Design review of the part built by this model. Coordinates are the model's own, in mm. Face numbers are marked on the shaded views. Round coordinates to 2 decimals unless told otherwise and drop trailing zeros. Order: outer loops, then holes, each group sorted by start corner. A loop starts at its lowest first (then second) coordinate and runs counter-clockwise, first axis right, second up. Notation, with made-up numbers: M 76.25,-32.5 L 113.25,-32.5 A30 cw 113.25,-1.5 Z; hole C 74,11 d1. An arc over 180 degrees is marked long. Write item = value, one per line. Start each with the question number.
```python
from build123d import *

# Parameters (mm, degrees)
F1_DEPTH = 2600
F2_W     = 560
F2_H     = 1279.0293264389
F3_DEPTH = 95.001
F4_W     = 765
F4_H     = 2300
F5_DEPTH = 95.001
F6_R     = 3


with BuildPart() as f1:
    # F0 (on Top) → F1 (new body)
    with BuildSketch(Plane.XY):
        Polygon((-271.6449069816, 555.1264761336), (-271.6449069816, -244.8735238664), (-176.6449069816, -244.8735238664), (-176.6449069816, 460.1264761336), (728.3550930184, 460.1264761336), (728.3550930184, 555.1264761336), align=None)
        Polygon((-259.1449069816, 542.6264761336), (715.8550930184, 542.6264761336), (715.8550930184, 472.6264761336), (-189.1449069816, 472.6264761336), (-189.1449069816, -232.3735238664), (-259.1449069816, -232.3735238664), align=None, mode=Mode.SUBTRACT)
    extrude(amount=F1_DEPTH)

    # F2 (on face) → F3 (cut, through all)
    with BuildSketch(Plane.YZ.offset(-176.6449069816)):
        with Locations((107.6264761336, 1660.4853367805)):
            Rectangle(F2_W, F2_H)
    extrude(amount=-F3_DEPTH, mode=Mode.SUBTRACT)

    # F4 (on face) → F5 (cut, through all)
    with BuildSketch(Plane.XZ.offset(-460.1264761336)):
        with Locations((275.8550930184, 1150)):
            Rectangle(F4_W, F4_H)
    extrude(amount=-F5_DEPTH, mode=Mode.SUBTRACT)

    # F6
    f6_edges = [f1.edges().sort_by_distance(p)[0] for p in [
        (-106.644907, 542.626476, 1150),
        (-106.644907, 548.876476, 0),
        (-106.644907, 555.126476, 1150),
        (-106.644907, 548.876476, 2300),
        (-106.644907, 460.126476, 1150),
        (-106.644907, 466.376476, 0),
        (-106.644907, 472.626476, 1150),
        (-106.644907, 466.376476, 2300),
        (275.855093, 542.626476, 2300),
        (275.855093, 555.126476, 2300),
        (658.355093, 548.876476, 2300),
        (275.855093, 460.126476, 2300),
        (275.855093, 472.626476, 2300),
        (658.355093, 466.376476, 2300),
        (-259.144907, 107.626476, 2300),
        (-265.394907, -172.373524, 2300),
        (-271.644907, 107.626476, 2300),
        (-265.394907, 387.626476, 2300),
        (-176.644907, 107.626476, 2300),
        (-182.894907, -172.373524, 2300),
        (-189.144907, 107.626476, 2300),
        (-182.894907, 387.626476, 2300),
        (-259.144907, 387.626476, 1660.485337),
        (-271.644907, 387.626476, 1660.485337),
        (-265.394907, 387.626476, 1020.970674),
        (-176.644907, 387.626476, 1660.485337),
        (-189.144907, 387.626476, 1660.485337),
        (-182.894907, 387.626476, 1020.970674),
        (-271.644907, -172.373524, 1660.485337),
        (-271.644907, 107.626476, 1020.970674),
        (658.355093, 555.126476, 1150),
        (-259.144907, -172.373524, 1660.485337),
        (-259.144907, 107.626476, 1020.970674),
        (658.355093, 542.626476, 1150),
        (-189.144907, -172.373524, 1660.485337),
        (-189.144907, 107.626476, 1020.970674),
        (658.355093, 472.626476, 1150),
        (658.355093, 460.126476, 1150),
        (-176.644907, 107.626476, 1020.970674),
        (-176.644907, -172.373524, 1660.485337),
    ]]
    fillet(f6_edges, radius=F6_R)


solid = f1.part
```
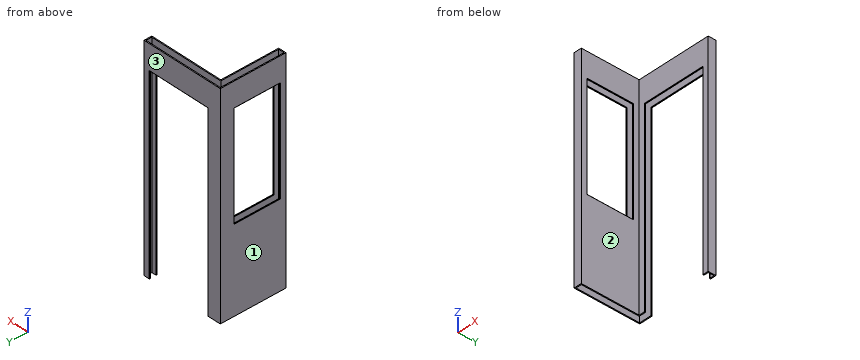
(1) Insertion check: pin 1 (2 mm diameter, centred on x = -265, y = 182.5, fed in from -Z); pin 2 (12 mm diameter, centred on y = 451.5, z = 1249, fed in from +X). Each pin has a flat end and moves straight along its axis. Give the tip position at first contact, or say it passes through.
(2) Consider section A-A, the plane x = -143. Write out the cut boundary in (y, z).
(3) For line 1 along Y through (x, z) = (-185.5, 1941); line 2 along Y through (x, z) = (636, 2445.5); line 3 along X through (y, z) = (483.5, 499), list the stretches that pass through material, from the lowest coordinate up. Write a range as [from, to].
(4) Consider section C-C, the plane z = 590.5. Write out the cut boundary in (x, y).
(5) Consider section B-B, the plane y = 161.5. Write out the cut boundary in (x, z).
(6) Draft analysis for pull direction X (two halves, no side actions). For the marked faces 1, 2 and 3, state which applies: pulls with the +X half, pulls with the -X half, needs draft (parallel to the pull), parting line crosses it, or undercut.
(7) Consider section D-D, the plane x = 426. Write out the cut boundary in (y, z), then the cut area to 3 significant figures.
Completed:
q1.pin_1 = 0
q1.pin_2 = -176.64
q2.outline = M 460.13,0 L 472.63,0 L 472.63,2600 L 460.13,2600 Z; M 542.63,0 L 555.13,0 L 555.13,2600 L 542.63,2600 Z
q3.line_1 = [-244.87, -172.37], [387.63, 472.63], [542.63, 555.13]
q3.line_2 = [460.13, 472.63], [542.63, 555.13]
q3.line_3 = [-271.64, -259.14], [715.86, 728.36]
q4.outline = M -271.64,-244.87 L -176.64,-244.87 L -176.64,460.13 L -109.64,460.13 A3 ccw -106.64,463.13 L -106.64,469.63 A3 ccw -109.64,472.63 L -189.14,472.63 L -189.14,-232.37 L -259.14,-232.37 L -259.14,542.63 L -109.64,542.63 A3 ccw -106.64,545.63 L -106.64,552.13 A3 ccw -109.64,555.13 L -271.64,555.13 Z; M 658.36,463.13 A3 ccw 661.36,460.13 L 728.36,460.13 L 728.36,555.13 L 661.36,555.13 A3 ccw 658.36,552.13 L 658.36,545.63 A3 ccw 661.36,542.63 L 715.86,542.63 L 715.86,472.63 L 661.36,472.63 A3 ccw 658.36,469.63 Z
q5.outline = M -271.64,0 L -259.14,0 L -259.14,1017.97 A3 ccw -262.14,1020.97 L -268.64,1020.97 A3 ccw -271.64,1017.97 Z; M -271.64,2303 A3 ccw -268.64,2300 L -262.14,2300 A3 ccw -259.14,2303 L -259.14,2600 L -271.64,2600 Z; M -189.14,0 L -176.64,0 L -176.64,1017.97 A3 ccw -179.64,1020.97 L -186.14,1020.97 A3 ccw -189.14,1017.97 Z; M -189.14,2303 A3 ccw -186.14,2300 L -179.64,2300 A3 ccw -176.64,2303 L -176.64,2600 L -189.14,2600 Z
q6.face_1 = pulls with the -X half
q6.face_2 = pulls with the +X half
q6.face_3 = needs draft
q7.outline = M 460.13,2303 A3 ccw 463.13,2300 L 469.63,2300 A3 ccw 472.63,2303 L 472.63,2600 L 460.13,2600 Z; M 542.63,2303 A3 ccw 545.63,2300 L 552.13,2300 A3 ccw 555.13,2303 L 555.13,2600 L 542.63,2600 Z
q7.area = 7,490 mm2
